Here's how the part is built. I have some questions about the finished solid (model axes, mm). A direction names the side the tool comes from. Give positions to 0.01 mm unless a question says otherwise; leave off trailing zeros. Write each loop counter-clockwise with the first axis right and the second up, starting at its lowest first coordinate (ties: lowest second). Pieces come first, ordered by that corner, then holes. Notation, with made-up numbers: (7.25, -27) - (63.25, -27) arc R19 cw to (63.25, 5) - close; hole circle Ø4 at (59.5, 48). An arc over 180 degrees is marked (long way). One line per item, written item: value. Start each with the question number.
1) We'd pull the mould along Z, two halves only. Please class faces 1 (the cylindrical face through (3.796, 1.676, -0.167)), 2 (the flat face through (0, 5, 0)), 3 (the cylindrical face through (1.17, 1.97, 5.27)): +Z half, -Z half, draft (parallel to the pull), parting line (faces both ways), or undercut.
2) Imagine slicing it at C-C on y = 0.95. Write out the boundary of the cut face in (x, z).
3) I'm going to push flat-ended pins straight in: P1, Ø1, axis at x = -3.5, z = 4, coming from the +Y side; P2, Ø4.5, axis at x = 0, z = 0, coming from the -Y side. Where does each tip first touch, or does it pass through?
4) On a 3-axis mill with a long thin cutter (end or side, diameter ignored), from which of +Z, -Z, +X, -X, +Y, -Y can I reach the whole of each face in a straight line? I mean faces 4 (the flat face through (-1, 0, 4)), 5 (the flat face through (0, 3.4, 0)). Say none if no direction works.
5) Imagine slicing it at A-A on x = 0. Write out the boundary of the cut face in (y, z).
6) Please list where these lines run through material, in increasing order: L1, parallel to Z at x = 0, y = 1.6; L2, parallel to Y at x = -2.5, z = 1; L3, parallel to X at y = 2.65, z = -1.25. Write a range as [from, to].
7) Imagine slicing it at B-B on z = 0. Write out the boundary of the cut face in (x, y), plus the area to 3 significant figures.
Autodesk Inventor part; units mm, degrees
ref_plane "YZ Plane" through (0, 0, 0) normal (1, 0, 0) x (0, 1, 0)
ref_plane "XZ Plane" through (0, 0, 0) normal (0, 1, 0) x (-1, 0, 0)
ref_plane "XY Plane" through (0, 0, 0) normal (0, 0, 1) x (1, 0, 0)
sketch "스케치1" plane through (0, 0, 0) normal (0, 1, 0) x (-1, 0, 0)
  circle A0 centre (0, 0) radius 3.8
  circle A1 centre (0, 0) radius 5.4
  dimension "d0" = 7.6
  dimension "d1" = 1.6
extrude "돌출1" add sketch "스케치1" along normal blind 5 contours A0 | A1
extrude "돌출2" cut sketch "스케치1" along normal blind 3.4 contours A0
fillet "모깎기1" radius 1 1 edges at (5.4, 5, 0)
properties part number "final_탄두낙하산거치대_스프링고정"
Numbers:
1. face 1: undercut
1. face 2: draft
1. face 3: parting line
2. outline: circle Ø10.8 at (0, 0); hole circle Ø7.6 at (0, 0)
3. P1: y = 4.91
3. P2: y = 3.4
4. face 4: +Z, -Z, +X, -X, -Y
4. face 5: -Y
5. outline: (0, -5.4) - (4, -5.4) arc R1 ccw to (5, -4.4) - (5, 4.4) arc R1 ccw to (4, 5.4) - (0, 5.4) - (0, 3.8) - (3.4, 3.8) - (3.4, -3.8) - (0, -3.8) - close
6. L1: [-5.4, -3.8], [3.8, 5.4]
6. L2: [3.4, 5]
6. L3: [-5.25, -3.59], [3.59, 5.25]
7. outline: (-5.4, 0) - (-3.8, 0) - (-3.8, 3.4) - (3.8, 3.4) - (3.8, 0) - (5.4, 0) - (5.4, 4) arc R1 ccw to (4.4, 5) - (-4.4, 5) arc R1 ccw to (-5.4, 4) - close
7. area: 27.7 mm^2
